from build123d import *

# Parameters (mm, degrees)
F1_DEPTH = 1
F3_DEPTH = 6
F4_R     = 1
F5_R     = 5
F7_DEPTH = 12.5
F8_SCALE = 1.2


# Not quite as in the source:
# - a feature names something its author has since deleted; it is built from what else it names


with BuildPart() as f1:
    # F0 (on Top) → F1 (new body)
    with BuildSketch(Plane.XY):
        Polygon((24, 30), (-24, 30), (-24, -20.3061967343), (-24, -30), (24, -30), (24, -20.3061967343), align=None)
        Polygon((-24, -30), (-24, -20.3061967343), (-26.5, -30), align=None)
        Polygon((26.5, -30), (24, -20.3061967343), (24, -30), align=None)
    extrude(amount=F1_DEPTH)

    # F2 (on face) → F3 (join)
    with BuildSketch(Plane.XY.offset(1)):
        with BuildLine():
            Line((24, 30), (24, -26.4028457212))
            ThreePointArc((24, -26.4028457212), (24.2165144832, -28.2514541736), (24.8543383025, -30))
            Line((24.8543383025, -30), (26.8543383025, -30))
            ThreePointArc((26.8543383025, -30), (26.2165144832, -28.2514541736), (26, -26.4028457212))
            Line((26, -26.4028457212), (26, 32))
            Line((26, 32), (0, 32))
            Line((0, 32), (-26, 32))
            Line((-26, 32), (-26, -26.4028457212))
            ThreePointArc((-26, -26.4028457212), (-26.2165144832, -28.2514541736), (-26.8543383025, -30))
            Line((-26.8543383025, -30), (-24.8543383025, -30))
            ThreePointArc((-24.8543383025, -30), (-24.2165144832, -28.2514541736), (-24, -26.4028457212))
            Line((-24, -26.4028457212), (-24, 30))
            Line((-24, 30), (0, 30))
            Line((0, 30), (24, 30))
        make_face()
    extrude(amount=-F3_DEPTH)

    # F4
    f4_edges = [f1.edges().sort_by_distance(p)[0] for p in [
        (-26.854338, -30, -2),
        (26.854338, -30, -2),
    ]]
    fillet(f4_edges, radius=F4_R)

    # F5
    f5_edges = [f1.edges().sort_by_distance(p)[0] for p in [
        (24, 30, -2.5),
        (26, 32, -2),
        (-26, 32, -2),
        (-24, 30, -2.5),
    ]]
    fillet(f5_edges, radius=F5_R)


with BuildPart() as f7:
    # F6 (on face) → F7 (new body, symmetric)
    with BuildSketch(Plane(origin=(0, 0, 0), x_dir=(1, 0, 0), z_dir=(0, 0, -1))):
        Polygon((6.3998643309, -23.389915917), (11.8633387856, -22.7571071915), (11.8633387856, 0), (6.3998643309, -0.6328087254), (6.3998643309, -10.9478783381), (6.3998643309, -13.2169965655), align=None)
        Polygon((-1.9300751453, -23.6877743155), (6.3998643309, -13.2169965655), (6.3998643309, -10.9478783381), (-1.1277758749, 0), (-6.5578306463, -0.8743598687), (0.8998643309, -11.7196280624), (-7.3682154656, -22.865199178), align=None)
    extrude(amount=F7_DEPTH, both=True)


with BuildPart() as f7_1:
    # F8: moved
    add(f7.part.scale(F8_SCALE))


with BuildPart() as f7_2:
    # F9: moved
    add(f7_1.part.moved(Location((-3.1, -0.5, 0))))


with BuildPart() as f1_1:
    add(f1.part)

    # F10: cut F7
    add(f7_2.part, mode=Mode.SUBTRACT)


solid = f1_1.part
Geometry: final body of the model. Coordinates: model frame, mm. A direction names the side the tool comes from. Round coordinates to 2 decimals unless told otherwise and drop trailing zeros. Write each loop counter-clockwise with the first axis right and the second up, starting at its lowest first coordinate (ties: lowest second). Pieces come first, ordered by that corner, then holes. Notation, with made-up numbers: M -19,-15.75 L 22,-15.75 A37 cw 22,22.25 Z; hole C 48.25,-4.75 d9. An arc over 180 degrees is marked long. Write item = value, one per line.
Item 1: Access query for faces 1 (the face through (-0.1, -30, 0.4)), 2 (the face through (23, 28, -3)), 3 (the face through (-6.912, 20.157, 0.493)). Directions: +Z, -Z, +X, -X, +Y, -Y. A direction counts if a zero-diameter tool reaches every point of the face in a straight line with its end or side. Return the directions, or none.
Findings:
face_1 = +Z, -Z, +X, -X, -Y
face_2 = -Z, -Y
face_3 = +Z, -Z
Item 2: Section query B-B on x = 0.5. Return loops of the section in (y, z).
Findings:
outline = M -30,0 L 6.7,0 L 6.7,1 L -30,1 Z; M 20.49,0 L 30,0 L 30,-5 L 32,-5 L 32,1 L 20.49,1 Z
Item 3: Section query D-D on y = -8. Return loops of the section in (x, z).
Findings:
outline = M -26,-5 L -24,-5 L -24,0 L 24,0 L 24,-5 L 26,-5 L 26,1 L -26,1 Z
Item 4: Section query C-C on y = 6. Return loops of the section in (x, z), then the cut area to 3 significant figures.
Findings:
outline = M -26,-5 L -24,-5 L -24,0 L -7.22,0 L -7.22,1 L -26,1 Z; M 0.02,0 L 4.58,0 L 4.58,1 L 0.02,1 Z; M 11.14,0 L 24,0 L 24,-5 L 26,-5 L 26,1 L 11.14,1 Z
area = 58.2 mm^2
Item 5: Pull-direction query (X, two-part tool) for faces 4 (the face through (0, 32, -2)), 5 (the face through (-24, -1, -2)), 6 (the face through (-24.223, -28.277, -2.465)), 7 (the face through (26, 0, -2)); classes: pulls with the +X half, pulls with the -X half, needs draft (parallel to the pull), parting line crosses it, or undercut.
Findings:
face_4 = needs draft
face_5 = undercut
face_6 = undercut
face_7 = pulls with the +X half
Item 6: Section query A-A on z = -2.85. Return loops of the section in (x, y).
Findings:
outline = M -26.34,-28.71 A1 ccw -25.38,-30 L -24.85,-30 A8 ccw -24,-26.4 L -24,25 A5 cw -19,30 L 19,30 A5 cw 24,25 L 24,-26.4 A8 ccw 24.85,-30 L 25.38,-30 A1 ccw 26.34,-28.71 A8 cw 26,-26.4 L 26,27 A5 ccw 21,32 L -21,32 A5 ccw -26,27 L -26,-26.4 A8 cw Z
Item 7: Material intervals for line 1 along X through (y, z) = (-20, -2.6); line 2 along Y through (x, z) = (-10.5, -0.6); line 3 along Z through (x, y) = (-16.5, -7), sorted ascending. Write a range as [from, to].
Findings:
line_1 = [-26, -24], [24, 26]
line_2 = [30, 32]
line_3 = [0, 1]
Item 8: Pin query (flat end, axial travel): P1, Ø2.5, axis at x = -5.5, z = -3, coming from the -Y side; P2, Ø1.5, axis at y = -2.5, z = -4.5, coming from the +X side; P3, Ø1.1, axis at y = 8.5, z = 0.5, coming from the -X side. Return the tip coordinate at first contact, or that it passes through.
Findings:
P1 = 30
P2 = 26
P3 = -26
